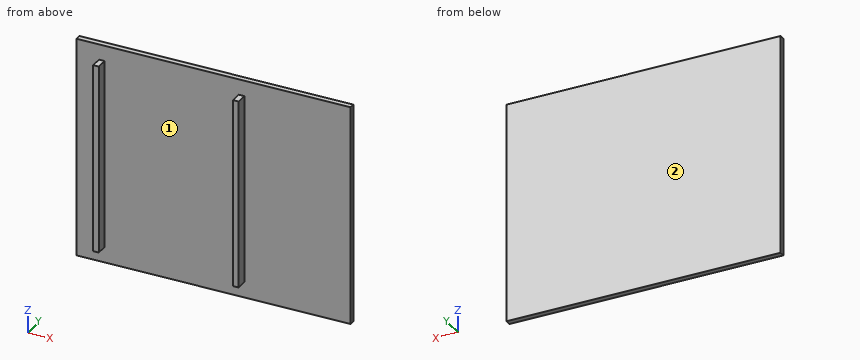
Autodesk Inventor part; units mm, degrees
ref_plane "YZ Plane" through (0, 0, 0) normal (1, 0, 0) x (0, 1, 0)
ref_plane "XZ Plane" through (0, 0, 0) normal (0, 1, 0) x (-1, 0, 0)
ref_plane "XY Plane" through (0, 0, 0) normal (0, 0, 1) x (1, 0, 0)
sketch "Sketch1" plane through (0, 0, 0) normal (0, 1, 0) x (-1, 0, 0)
  line L0 (0, 0) -> (-155.575, 0)
  line L1 (-155.575, 0) -> (-155.575, 125.73)
  line L2 (-155.575, 125.73) -> (0, 125.73)
  line L3 (0, 125.73) -> (0, 0)
  dimension "d0" = 155.575
  dimension "d1" = 125.73
extrude "Extrusion1" add sketch "Sketch1" along normal blind 3.175
sketch "Sketch2" plane through (0, 0, 0) normal (0, -1, 0) x (1, 0, 0)
  line L0 (155.575, 0) -> (0, 0) construction
  line L1 (0, 0) -> (12.7, 0) construction
  line L2 (0, 125.73) -> (155.575, 125.73) construction
  line L3 (12.7, 0) -> (15.875, 0) construction
  line L4 (15.875, 0) -> (15.875, 125.73) construction
  line L5 (15.875, 125.73) -> (12.7, 125.73) construction
  line L6 (12.7, 125.73) -> (12.7, 0) construction
  line L7 (15.875, 0) -> (92.075, 0) construction
  line L8 (23.8468, 0) -> (23.8468, 8.89) construction
  line L9 (23.8468, 125.73) -> (23.8468, 116.84) construction
  line L10 (23.8468, 8.89) -> (15.875, 8.89) construction
  line L11 (23.8468, 116.84) -> (15.875, 116.84) construction
  line L12 (92.075, 0) -> (92.075, 125.73) construction
  line L13 (23.8468, 116.84) -> (92.075, 116.84) construction
  line L14 (23.8468, 8.89) -> (92.075, 8.89) construction
  line L15 (15.875, 8.89) -> (12.7, 8.89)
  line L16 (12.7, 8.89) -> (12.7, 116.84)
  line L17 (12.7, 116.84) -> (15.875, 116.84)
  line L18 (15.875, 116.84) -> (15.875, 8.89)
  line L19 (92.075, 8.89) -> (95.25, 8.89)
  line L20 (95.25, 8.89) -> (95.25, 116.84)
  line L21 (95.25, 116.84) -> (92.075, 116.84)
  line L22 (92.075, 116.84) -> (92.075, 8.89)
  dimension "d4" = 12.7
  dimension "d5" = 3.175
  dimension "d6" = 76.2
  dimension "d11" = 8.89
  dimension "d12" = 8.89
  dimension "d13" = 3.175
  dimension "d14" = 107.95
extrude "Extrusion2" add sketch "Sketch2" along normal blind 6.35
properties part number "False_Bottom"
The model under review builds one solid part; all positions refer to its coordinate system, in mm. Face numbers are marked on the shaded views. Give positions to 0.01 mm unless a question says otherwise; leave off trailing zeros. Write each loop counter-clockwise with the first axis right and the second up, starting at its lowest first coordinate (ties: lowest second). Pieces come first, ordered by that corner, then holes. Notation, with made-up numbers: M -38,-23.75 L 20,-23.75 A22 cw 20,-3.75 Z; hole C -1,40 d11. An arc over 180 degrees is marked long. Write item = value, one per line. Start each with the question number.
Q1. We need section C-C (x = 31). State the section outline as (y, z) points (3 decimals), plus the area to 3 significant figures.
Q2. Clearance check with flat-ended pins moving along their axes: pin 1 (1.6 mm diameter, centred on x = 15, y = -3.5, fed in from +Z); pin 2 (5 mm diameter, centred on y = -3.5, z = 39.5, fed in from -X); pin 3 (2.5 mm diameter, centred on x = 14.5, y = -3, fed in from -Z). State where each tip first meets the part, or that it passes through.
Q3. We need section A-A (y = -4.25). State the section outline as (x, z) points (3 decimals).
Q4. We need section B-B (z = 21.5). State the section outline as (x, y) points (3 decimals), plus the area to 3 significant figures.
Q5. Mouldability with a two-part tool opening along X and no side actions: class the marked faces 1 and 2 as released by +X, released by -X, zero draft, split by the parting line, or undercut.
Q6. For line 1 (X direction, y = -2.5, z = 116.5) (3 decimals); line 2 (Y direction, x = 58, z = 94.5) (3 decimals), list the stretches that pass through material, from the lowest coordinate up.
Result set:
q1.outline = M 0,0 L 3.175,0 L 3.175,125.73 L 0,125.73 Z
q1.area = 399 mm2
q2.pin_1 = 116.84
q2.pin_2 = 12.7
q2.pin_3 = 8.89
q3.outline = M 12.7,8.89 L 15.875,8.89 L 15.875,116.84 L 12.7,116.84 Z; M 92.075,8.89 L 95.25,8.89 L 95.25,116.84 L 92.075,116.84 Z
q4.outline = M 0,0 L 12.7,0 L 12.7,-6.35 L 15.875,-6.35 L 15.875,0 L 92.075,0 L 92.075,-6.35 L 95.25,-6.35 L 95.25,0 L 155.575,0 L 155.575,3.175 L 0,3.175 Z
q4.area = 534 mm2
q5.face_1 = undercut
q5.face_2 = zero draft
q6.line_1 = 12.7 to 15.875, 92.075 to 95.25
q6.line_2 = 0 to 3.175
